```python
from build123d import *

# Parameters (mm, degrees)
SKETCH1_R           = 5.9
SKETCH1_R_2         = 2.3
BOSS_EXTRUDE1_DEPTH = 5
SKETCH2_W           = 42.9
SKETCH2_H           = 14.13586664
BOSS_EXTRUDE2_DEPTH = 5
SKETCH3_W           = 14.13586664
SKETCH3_H           = 13.416162411
BOSS_EXTRUDE3_DEPTH = 5


with BuildPart() as part:
    # Sketch1 → Boss-Extrude1 (new body)
    with BuildSketch(Plane(origin=(0, 0, 0), x_dir=(1, 0, 0), z_dir=(0, 1, 0))):
        with Locations(Location((0, 0, 0), (0, 0, 270))):
            Circle(SKETCH1_R)
        with Locations(Location((0, 0, 0), (0, 0, 270))):
            Circle(SKETCH1_R_2, mode=Mode.SUBTRACT)
    extrude(amount=BOSS_EXTRUDE1_DEPTH)

    # Sketch2 → Boss-Extrude2 (add)
    with BuildSketch(Plane(origin=(0, 5, 0), x_dir=(1, 0, 0), z_dir=(0, 1, 0))):
        Rectangle(SKETCH2_W, SKETCH2_H)
    extrude(amount=BOSS_EXTRUDE2_DEPTH)

    # Sketch3 → Boss-Extrude3 (add)
    with BuildSketch(Plane.ZY.offset(21.45)):
        with Locations((0, 11.708081206)):
            Rectangle(SKETCH3_W, SKETCH3_H)
    boss_extrude3 = extrude(amount=BOSS_EXTRUDE3_DEPTH)

    # Mirror1: Boss-Extrude3 across plane
    add(boss_extrude3.mirror(Plane(origin=(0, 0, 0), x_dir=(0, 0, 1), z_dir=(1, 0, 0))))


solid = part.part
```
Read the model definition and answer for the solid it produces. Units are mm, in the model's axes. A direction names the side the tool comes from. Give positions to 0.01 mm unless a question says otherwise; leave off trailing zeros. Order: outer loops, then holes, each group sorted by start corner. A loop starts at its lowest first (then second) coordinate and runs counter-clockwise, first axis right, second up.
(1) Find section C-C (x = 0). Give the vertices of the cut face in (y, z), plus the area to 3 significant figures.
(2) Given pin 1 (1.5 mm diameter, centred on x = -6.5, z = 3, fed in from -Y); pin 2 (1 mm diameter, centred on x = -15, z = 1, fed in from +Y), each flat-ended and moving along its own axis, determine where each tip first touches the part or whether it passes through.
(3) For faces 1 (the flat face through (0, 10, 0)), 2 (the flat face through (0, 5, 0)), 3 (the flat face through (-24, 18.416, 0)), determine the directions among +Z, -Z, +X, -X, +Y, -Y from which every point of the face is accessible in a straight line to the end or side of a thin tool.
(4) Find section A-A (y = 16.25). Give the vertices of the cut face in (x, z), plus the area to 3 significant figures.
(5) Find section B-B (z = 0). Give the vertices of the cut face in (x, y).
(6) For a pull along X with two mould halves and no side action, classify faces 4 (the flat face through (21.45, 14, 0)), 5 (the cylindrical face through (0.691, 2.465, 2.194)), 6 (the flat face through (26.45, 12, 0)), 7 (the flat face through (0, 9, -7.068)) as released by +X, released by -X, zero draft, split by the parting line, or undercut.
(7) Find section D-D (z = 3). Give the vertices of the cut face in (x, y), plus the area to 3 significant figures.
(8) Straight lines are drawn through the part: L1, parallel to X at y = 14, z = 4.75; L2, parallel to X at y = 2.15, z = 0; L3, parallel to Y at x = -2, z = 2. For each, find the intervals that lie inside material, in ascending order.
Result sheet:
1. outline: (0, -5.9) - (5, -5.9) - (5, -7.07) - (10, -7.07) - (10, 7.07) - (5, 7.07) - (5, 5.9) - (0, 5.9) - (0, 2.3) - (5, 2.3) - (5, -2.3) - (0, -2.3) - close
1. area: 107 mm2
2. pin 1: stops at y = 5
2. pin 2: stops at y = 10
3. face 1: +Z, -Z, +Y
3. face 2: -Y
3. face 3: +Z, -Z, +X, -X, +Y
4. outline: (-26.45, -7.07) - (-21.45, -7.07) - (-21.45, 7.07) - (-26.45, 7.07) - close; (21.45, -7.07) - (26.45, -7.07) - (26.45, 7.07) - (21.45, 7.07) - close
4. area: 141 mm2
5. outline: (-26.45, 5) - (-5.9, 5) - (-5.9, 0) - (-2.3, 0) - (-2.3, 5) - (2.3, 5) - (2.3, 0) - (5.9, 0) - (5.9, 5) - (26.45, 5) - (26.45, 18.42) - (21.45, 18.42) - (21.45, 10) - (-21.45, 10) - (-21.45, 18.42) - (-26.45, 18.42) - close
6. face 4: undercut
6. face 5: undercut
6. face 6: released by +X
6. face 7: zero draft
7. outline: (-26.45, 5) - (-5.08, 5) - (-5.08, 0) - (5.08, 0) - (5.08, 5) - (26.45, 5) - (26.45, 18.42) - (21.45, 18.42) - (21.45, 10) - (-21.45, 10) - (-21.45, 18.42) - (-26.45, 18.42) - close
7. area: 399 mm2
8. L1: x = -26.45 to -21.45, 21.45 to 26.45
8. L2: x = -5.9 to -2.3, 2.3 to 5.9
8. L3: y = 0 to 10
